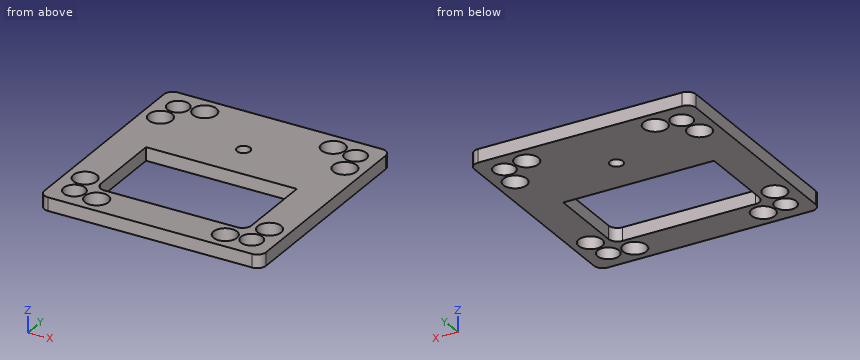
Autodesk Inventor part; units mm, degrees
ref_plane "YZ Plane" through (0, 0, 0) normal (1, 0, 0) x (0, 1, 0)
ref_plane "XZ Plane" through (0, 0, 0) normal (0, 1, 0) x (-1, 0, 0)
ref_plane "XY Plane" through (0, 0, 0) normal (0, 0, 1) x (1, 0, 0)
sketch "Skizze1" plane through (0, 0, 0) normal (0, 0, 1) x (1, 0, 0)
  line L0 (-17.4, -0.2) -> (-25.4, -0.2)
  line L1 (-25.4, -0.2) -> (-25.4, -23.2)
  line L2 (-23.4, -25.2) -> (-0.4, -25.2)
  line L3 (-0.4, -25.2) -> (-0.4, -17.2)
  line L4 (-17.4, -0.2) -> (-17.4, -15.2)
  line L5 (-15.4, -17.2) -> (-0.4, -17.2)
  arc A0 (-25.4, -23.2) -> (-23.4, -25.2) centre (-23.4, -23.2) ccw
  circle A1 centre (-20.4, -20.2) radius 2.425
  circle A2 centre (-21.2, -14.7) radius 2.65
  circle A3 centre (-14.9, -21) radius 2.65
  arc A4 (-17.4, -15.2) -> (-15.4, -17.2) centre (-15.4, -15.2) ccw
  circle A5 centre (-20.4, -20.2) radius 2.425
  circle A6 centre (-14.9, -21) radius 2.65
  circle A7 centre (-21.2, -14.7) radius 2.65
  point P0 (-25.4, -25.2)
  point P1 (-17.4, -17.2)
  dimension "d278" = 25
  dimension "d279" = 25
  dimension "d2" = 8
  dimension "d281" = 8
  dimension "d282" = 2
  dimension "d283" = 4.85
  dimension "d284" = 20
  dimension "d4" = 20
  dimension "d286" = 5.3
  dimension "d_hole" = 5.3
  dimension "d290" = 20.8
  dimension "d" = 20.8
  dimension "d292" = 2
  dimension "d313" = 6.3
  dimension "d314" = 6.3
  dimension "d330" = 0
  dimension "d331" = 0
  dimension "d332" = 0
extrude "Extrusion1" add sketch "Skizze1" along normal blind 3
mirror "Mirror6" about plane through (-17.4, -0.2, 0) normal (0, 1, 0) of "Extrusion1"
mirror "Mirror7" about plane through (-0.4, -25.2, 0) normal (1, 0, 0) of "Extrusion1", "Mirror6"
sketch "Sketch32" plane through (0, 0, 3) normal (0, 0, 1) x (1, 0, 0)
  circle A0 centre (-0.54, 11.03) radius 1.4
  circle A1 centre (-0.54, 11.03) radius 7 construction
  circle A2 centre (-0.54, 11.03) radius 1.75
  line L0 (22.6, 24.8) -> (-23.4, 24.8)
  arc A3 (-23.4, 24.8) -> (-25.4, 22.8) centre (-23.4, 22.8) ccw
  line L1 (-25.4, -23.2) -> (-25.4, 22.8)
  arc A4 (-25.4, -23.2) -> (-23.4, -25.2) centre (-23.4, -23.2) ccw
  line L2 (-23.4, -25.2) -> (22.6, -25.2)
  arc A5 (22.6, -25.2) -> (24.6, -23.2) centre (22.6, -23.2) ccw
  line L3 (24.6, 22.8) -> (24.6, -23.2)
  arc A6 (24.6, 22.8) -> (22.6, 24.8) centre (22.6, 22.8) ccw
  circle A7 centre (19.6, 19.8) radius 2.425
  circle A8 centre (14.1, 20.6) radius 2.65
  circle A9 centre (20.4, 14.3) radius 2.65
  circle A10 centre (19.6, -20.2) radius 2.425
  circle A11 centre (14.1, -21) radius 2.65
  circle A12 centre (20.4, -14.7) radius 2.65
  circle A13 centre (-20.4, 19.8) radius 2.425
  circle A14 centre (-14.9, 20.6) radius 2.65
  circle A15 centre (-21.2, 14.3) radius 2.65
  circle A16 centre (-21.2, -14.7) radius 2.65
  circle A17 centre (-14.9, -21) radius 2.65
  circle A18 centre (-20.4, -20.2) radius 2.425
  line L4 (14.6, 16.8) -> (-15.4, 16.8)
  arc A19 (16.6, 14.8) -> (14.6, 16.8) centre (14.6, 14.8) ccw
  line L5 (16.6, 14.8) -> (16.6, -15.2)
  arc A20 (14.6, -17.2) -> (16.6, -15.2) centre (14.6, -15.2) ccw
  line L6 (-15.4, -17.2) -> (14.6, -17.2)
  arc A21 (-17.4, -15.2) -> (-15.4, -17.2) centre (-15.4, -15.2) ccw
  line L7 (-17.4, -15.2) -> (-17.4, 14.8)
  arc A22 (-15.4, 16.8) -> (-17.4, 14.8) centre (-15.4, 14.8) ccw
  line L8 (16.6, 14.8) -> (16.6, -15.2)
  circle A23 centre (-0.54, 11.03) radius 1.5
  line L9 (16.6, 2.2667) -> (-17.4, 2.2667)
  line L10 (-17.4, -15.2) -> (-17.4, 14.8)
  point P0 (0, 0)
  dimension "d354" = 3
extrude "Extrusion17" add sketch "Sketch32" against normal blind 3 contours A2 | A19 L5 L9 L7 A22 L4
equation "\"d_i\" = 40"
equation "\"d_o\" = 40"
equation "\"d_part\" = 50"
equation "\"d6\" = 0"
equation "\"d7\" = 0"
equation "\"d8\" = 0"
equation "\"d9\" = 0"
equation "\"d13\" = 0"
equation "\"d14\" = 0"
equation "\"d20\" = 0"
equation "\"d21\" = 0"
equation "\"d22\" = 0"
equation "\"d23\" = 0"
equation "\"d24\" = 0"
equation "\"d25\" = 3"
equation "\"d26\" = 0"
equation "\"d27\" = 0"
equation "\"d28\" = 0"
equation "\"d29\" = 0"
equation "\"d30\" = 0"
equation "\"d31\" = 0"
equation "\"d32\" = 0"
equation "\"d33\" = 0"
equation "\"d34\" = 0"
equation "\"d46\" = 0"
equation "\"d47\" = 0"
equation "\"d48\" = 0"
equation "\"d50\" = 0"
equation "\"d51\" = 0"
equation "\"d52\" = 0"
equation "\"d53\" = 0"
equation "\"d54\" = 0"
equation "\"d55\" = 0"
equation "\"d56\" = 0"
equation "\"d57\" = 0"
equation "\"d58\" = 0"
equation "\"d59\" = 0"
equation "\"magnet_offset\" = 0"
equation "\"screw_offset\" = 0"
equation "\"mal_puzzle_offset\" = 0"
equation "\"fem_puzzle_offset\" = 0"
properties part number "30_Cube_Z_Focus_MGN_NEMA_counterplate"
Model file for the job. Use its own axes, mm. Coordinates: 2 decimals unless noted, no trailing zeros. Loops run counter-clockwise (first coordinate to the right, second up) from the corner with the lowest first, then second, coordinate; pieces in that order, holes last. Notation, with made-up numbers: M 87.25,30.25 L 115.25,30.25 A24 cw 115.25,43.25 Z; hole C 14,68 d10. An arc over 180 degrees is marked long. Use CSV: the item, a comma, the result in double quotes. Start each with the question number.
1. Band-saw the part on D-D, the plane x = -21.2. List the corners of the cut face in (y, z), then the cut area to 3 significant figures.
2. Flat gauge pin, fed straight in: pin 1 (4 mm diameter, centred on x = 19.6, y = 19.8, fed in from -Z). Where does the tip first touch, or does it go through?
3. Band-saw the part on B-B, the plane z = 2.25. Give the number of separate pieces and of enclosed holes in the cut face, then the cut area to 3 significant figures.
4. Probe probe 1 along X at (y, z) = (-14.5, 1.05); probe 2 along Y at (x, z) = (-20.4, 1.75) (3 decimals); probe 3 along Y at (x, z) = (-9.5, 0.9). List the from-to ranges inside material, lowest first. Write a range as [from, to].
5. Band-saw the part on A-A, the plane x = -0.54. List the corners of the cut face in (y, z), then the cut area to 3 significant figures.
6. Band-saw the part on C-C, the plane y = -20.2. List the corners of the cut face in (x, z) (3 decimals), then the cut area to 3 significant figures.
Entries:
1,outline,"M -25.2,0 L -22.49,0 L -22.49,3 L -25.2,3 Z; M -17.91,0 L -17.35,0 L -17.35,3 L -17.91,3 Z; M -12.05,0 L 11.65,0 L 11.65,3 L -12.05,3 Z; M 16.95,0 L 17.51,0 L 17.51,3 L 16.95,3 Z; M 22.09,0 L 24.8,0 L 24.8,3 L 22.09,3 Z"
1,area,"90.7 mm2"
2,pin 1,"passes through"
3,separate pieces,"1"
3,enclosed holes,"14"
3,area,"1,580 mm2"
4,probe 1,"x = [-25.4, -23.84], [-18.56, -17.4], [16.6, 17.76], [23.04, 24.6]"
4,probe 2,"y = [-25.2, -22.625], [-17.775, -17.226], [-12.174, 11.774], [16.826, 17.375], [22.225, 24.8]"
4,probe 3,"y = [-25.2, -17.2], [2.27, 24.8]"
5,outline,"M -25.2,0 L -17.2,0 L -17.2,3 L -25.2,3 Z; M 2.27,0 L 9.53,0 L 9.53,3 L 2.27,3 Z; M 12.53,0 L 24.8,0 L 24.8,3 L 12.53,3 Z"
5,area,"82.6 mm2"
6,outline,"M -25.4,0 L -22.825,0 L -22.825,3 L -25.4,3 Z; M -17.975,0 L -17.426,0 L -17.426,3 L -17.975,3 Z; M -12.374,0 L 11.574,0 L 11.574,3 L -12.374,3 Z; M 16.626,0 L 17.175,0 L 17.175,3 L 16.626,3 Z; M 22.025,0 L 24.6,0 L 24.6,3 L 22.025,3 Z"
6,area,"90.6 mm2"
